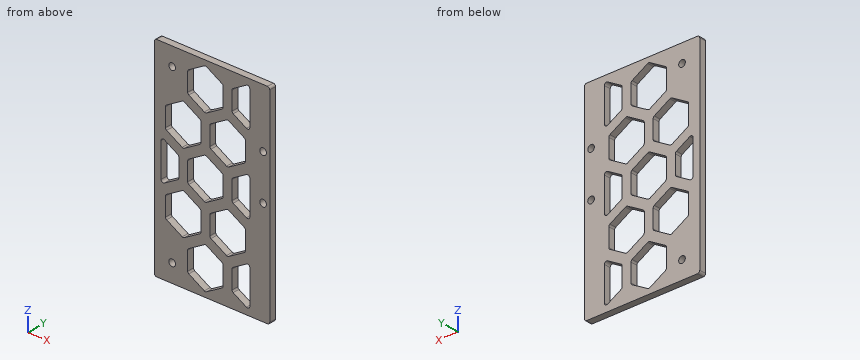
```python
from build123d import *

# Parameters (mm, degrees)
SKETCH_1_W          = 52
SKETCH_1_H          = 92
SKETCH_1_R          = 1.5
EXTRUDE_1_DEPTH     = 3
FILLET_1_R          = 1
CUT_EXTRUDE_1_DEPTH = 10
FILLET_2_R          = 1


with BuildPart() as part:
    # 草图1 → 凸台-拉伸1 (new body)
    with BuildSketch(Plane(origin=(0, 0, 0), x_dir=(1, 0, 0), z_dir=(0, 1, 0))):
        with Locations((26, 46)):
            Rectangle(SKETCH_1_W, SKETCH_1_H)
        with Locations(Location((49, 46, 0), (0, 0, 270))):
            Circle(SKETCH_1_R, mode=Mode.SUBTRACT)
        with Locations(Location((49, 26, 0), (0, 0, 270))):
            Circle(SKETCH_1_R, mode=Mode.SUBTRACT)
        with Locations(Location((8, 84, 0), (0, 0, 270))):
            Circle(SKETCH_1_R, mode=Mode.SUBTRACT)
        with Locations(Location((8, 8, 0), (0, 0, 270))):
            Circle(SKETCH_1_R, mode=Mode.SUBTRACT)
    extrude(amount=EXTRUDE_1_DEPTH)

    # 圆角1
    fillet_1_edges = [part.edges().sort_by_distance(p)[0] for p in [
        (0, 1.5, -92),
        (52, 1.5, -92),
        (52, 1.5, 0),
        (0, 1.5, 0),
    ]]
    fillet(fillet_1_edges, radius=FILLET_1_R)

    # 草图2 → 切除-拉伸1 (cut)
    with BuildSketch(Plane(origin=(0, 3, 0), x_dir=(1, 0, 0), z_dir=(0, 1, 0))):
        Polygon((23, 89.878620458), (15, 85.259818305), (15, 76.022213998), (23, 71.403411844), (31, 76.022213998), (31, 85.259818305), align=None)
        Polygon((13, 72.558112383), (5, 67.939310229), (5, 58.701705922), (13, 54.082903769), (21, 58.701705922), (21, 67.939310229), align=None)
        Polygon((43, 89.878620458), (35, 85.259818305), (35, 76.022213998), (43, 71.403411844), align=None)
        Polygon((23, 55.237604307), (15, 50.618802154), (15, 41.381197846), (23, 36.762395693), (31, 41.381197846), (31, 50.618802154), align=None)
        Polygon((3, 36.762395693), (11, 41.381197846), (11, 50.618802154), (3, 55.237604307), align=None)
        Polygon((35, 50.618802154), (43, 55.237604307), (43, 36.762395693), (35, 41.381197846), align=None)
        Polygon((25, 67.939310229), (33, 72.558112383), (41, 67.939310229), (41, 58.701705922), (33, 54.082903769), (25, 58.701705922), align=None)
        Polygon((21, 24.060689771), (13, 19.441887617), (5, 24.060689771), (5, 33.298294078), (13, 37.917096231), (21, 33.298294078), align=None)
        Polygon((25, 33.298294078), (25, 24.060689771), (33, 19.441887617), (41, 24.060689771), (41, 33.298294078), (33, 37.917096231), align=None)
        Polygon((43, 2.121379542), (35, 6.740181695), (35, 15.977786002), (43, 20.596588156), align=None)
        Polygon((31, 6.740181695), (23, 2.121379542), (15, 6.740181695), (15, 15.977786002), (23, 20.596588156), (31, 15.977786002), align=None)
    extrude(amount=-CUT_EXTRUDE_1_DEPTH, mode=Mode.SUBTRACT)

    # 圆角2
    fillet_2_edges = [part.edges().sort_by_distance(p)[0] for p in [
        (23, 1.5, -55.237604307),
        (31, 1.5, -50.618802154),
        (31, 1.5, -41.381197846),
        (23, 1.5, -36.762395693),
        (15, 1.5, -41.381197846),
        (15, 1.5, -50.618802154),
        (25, 1.5, -58.701705922),
        (25, 1.5, -67.939310229),
        (33, 1.5, -72.558112383),
        (41, 1.5, -67.939310229),
        (41, 1.5, -58.701705922),
        (33, 1.5, -54.082903769),
        (3, 1.5, -36.762395693),
        (3, 1.5, -55.237604307),
        (11, 1.5, -50.618802154),
        (11, 1.5, -41.381197846),
        (25, 1.5, -33.298294078),
        (33, 1.5, -37.917096231),
        (41, 1.5, -33.298294078),
        (41, 1.5, -24.060689771),
        (33, 1.5, -19.441887617),
        (25, 1.5, -24.060689771),
        (13, 1.5, -72.558112383),
        (21, 1.5, -67.939310229),
        (21, 1.5, -58.701705922),
        (13, 1.5, -54.082903769),
        (5, 1.5, -58.701705922),
        (5, 1.5, -67.939310229),
        (43, 1.5, -89.878620458),
        (43, 1.5, -71.403411844),
        (35, 1.5, -76.022213998),
        (35, 1.5, -85.259818305),
        (21, 1.5, -33.298294078),
        (21, 1.5, -24.060689771),
        (13, 1.5, -19.441887617),
        (5, 1.5, -24.060689771),
        (5, 1.5, -33.298294078),
        (13, 1.5, -37.917096231),
        (35, 1.5, -41.381197846),
        (35, 1.5, -50.618802154),
        (43, 1.5, -55.237604307),
        (43, 1.5, -36.762395693),
        (43, 1.5, -20.596588156),
        (43, 1.5, -2.121379542),
        (35, 1.5, -6.740181695),
        (35, 1.5, -15.977786002),
        (31, 1.5, -15.977786002),
        (31, 1.5, -6.740181695),
        (23, 1.5, -2.121379542),
        (15, 1.5, -6.740181695),
        (15, 1.5, -15.977786002),
        (23, 1.5, -20.596588156),
        (23, 1.5, -89.878620458),
        (31, 1.5, -85.259818305),
        (31, 1.5, -76.022213998),
        (23, 1.5, -71.403411844),
        (15, 1.5, -76.022213998),
        (15, 1.5, -85.259818305),
    ]]
    fillet(fillet_2_edges, radius=FILLET_2_R)


solid = part.part
```
Build history of the part. All positions in model axes, mm. Give positions to 0.01 mm unless a question says otherwise; leave off trailing zeros. Loops run counter-clockwise (first coordinate to the right, second up) from the corner with the lowest first, then second, coordinate; pieces in that order, holes last. Notation, with made-up numbers: (23.5, 30) -> (56.5, 30) arc R18 cw to (56.5, 65) -> close; hole circle Ø6 at (-7.75, -25.5). An arc over 180 degrees is marked (long way). One line per question, with ' | ' between items. Start each with the question number.
1) Cut at A-A (z = -46). Give the cut face in (x, y).
2) Probe L1, parallel to X at y = 1.15, z = -26; L2, parallel to X at y = 0.1, z = -28; L3, parallel to Z at x = 24.5, y = 1.05. List the from-to ranges inside material, lowest first.
3) Cut at B-B (x = 49). Give the cut face in (y, z), plus the area to 3 significant figures.
4) Cut at D-D (x = 39). Give the cut face in (y, z), plus the area to 3 significant figures.
5) Cut at C-C (z = -26). Give the cut face in (x, y), plus the area to 3 significant figures.
Return value:
1) outline: (0, 0) -> (3, 0) -> (3, 3) -> (0, 3) -> close; (11, 0) -> (15, 0) -> (15, 3) -> (11, 3) -> close; (31, 0) -> (35, 0) -> (35, 3) -> (31, 3) -> close; (43, 0) -> (47.5, 0) -> (47.5, 3) -> (43, 3) -> close; (50.5, 0) -> (52, 0) -> (52, 3) -> (50.5, 3) -> close
2) L1: 0 to 5, 21 to 25, 41 to 47.5, 50.5 to 52 | L2: 0 to 5, 21 to 25, 41 to 52 | L3: -92 to -89.01, -72.27 to -54.37, -37.63 to -19.73, -2.99 to 0
3) outline: (0, -92) -> (3, -92) -> (3, -47.5) -> (0, -47.5) -> close; (0, -44.5) -> (3, -44.5) -> (3, -27.5) -> (0, -27.5) -> close; (0, -24.5) -> (3, -24.5) -> (3, 0) -> (0, 0) -> close | area: 258 mm^2
4) outline: (0, -92) -> (3, -92) -> (3, -87.57) -> (0, -87.57) -> close; (0, -73.71) -> (3, -73.71) -> (3, -69.09) -> (0, -69.09) -> close; (0, -57.55) -> (3, -57.55) -> (3, -52.93) -> (0, -52.93) -> close; (0, -39.07) -> (3, -39.07) -> (3, -34.45) -> (0, -34.45) -> close; (0, -22.91) -> (3, -22.91) -> (3, -18.29) -> (0, -18.29) -> close; (0, -4.43) -> (3, -4.43) -> (3, 0) -> (0, 0) -> close | area: 82.0 mm^2
5) outline: (0, 0) -> (5, 0) -> (5, 3) -> (0, 3) -> close; (21, 0) -> (25, 0) -> (25, 3) -> (21, 3) -> close; (41, 0) -> (47.5, 0) -> (47.5, 3) -> (41, 3) -> close; (50.5, 0) -> (52, 0) -> (52, 3) -> (50.5, 3) -> close | area: 51.0 mm^2
